Autodesk Inventor part; units mm, degrees
ref_plane "YZ Plane" through (0, 0, 0) normal (1, 0, 0) x (0, 1, 0)
ref_plane "XZ Plane" through (0, 0, 0) normal (0, 1, 0) x (-1, 0, 0)
ref_plane "XY Plane" through (0, 0, 0) normal (0, 0, 1) x (1, 0, 0)
sketch "スケッチ1" plane through (0, 0, 0) normal (0, 1, 0) x (-1, 0, 0)
  line L0 (-13.5, 21) -> (-19.5, 21)
  line L1 (-19.5, 21) -> (-19.5, 0)
  line L2 (-19.5, 0) -> (19.5, 0)
  line L3 (19.5, 0) -> (19.5, 21)
  line L4 (19.5, 21) -> (13.5, 21)
  line L5 (13.5, 21) -> (13.5, 47)
  line L6 (13.5, 47) -> (19.5, 47)
  line L7 (19.5, 47) -> (19.5, 53)
  line L8 (19.5, 53) -> (-19.5, 53)
  line L9 (-19.5, 53) -> (-19.5, 47)
  line L10 (-19.5, 47) -> (-13.5, 47)
  line L11 (-13.5, 47) -> (-13.5, 21)
  point P0 (0, 0)
  point P1 (0, 0)
  dimension "d5" = 39
  dimension "d6" = 27
  dimension "d8" = 26
  dimension "d16" = 6
  dimension "d43" = 53
  dimension "d44" = 39
extrude "Body" add sketch "スケッチ1" along normal blind 0.8
fillet "フィレット1" radius 1 6 edges at (19.5, 0.4, 53) (19.5, 0.4, 47) (19.5, 0.4, 21) (-19.5, 0.4, 21) (-19.5, 0.4, 53) (-19.5, 0.4, 47)
sketch "スケッチ6" plane through (0, 0, 0) normal (0, -1, 0) x (1, 0, 0)
  circle A0 centre (0, 18.2) radius 7.5
  line L0 (19.5, 0) -> (-19.5, 0)
  circle A1 centre (0, 18.2) radius 10
  point P0 (0, 0)
  point P1 (0, 0)
  dimension "d27" = 15
  dimension "d28" = 20
  dimension "d31" = 18.2
extrude "押し出し4" cut sketch "スケッチ6" against normal through all contours A0
sketch "スケッチ7" plane through (0, 0.8, 0) normal (0, 1, 0) x (1, 0, 0)
  spline S0 degree 5 poles (0, 0) (-0.3117, -0.0168) (-0.9317, -0.0488) (-1.8515, -0.0923) (-3.0577, -0.1409) (-4.5307, -0.1873) (-5.9672, -0.223) (-7.3645, -0.2562) (-8.7185, -0.3001) (-10.0237, -0.3761) (-11.2732, -0.5129) (-12.4592, -0.7408) (-13.5734, -1.0876) (-14.6076, -1.5729) (-15.5546, -2.2027) (-16.4082, -2.9673) (-17.1633, -3.8489) (-17.8162, -4.8254) (-18.3648, -5.8755) (-18.8088, -6.9843) (-19.1492, -8.1424) (-19.3399, -9.1044) (-19.4375, -9.8448) (-19.4825, -10.3469) (-19.5, -10.6) knots 0 0 0 0 0 0 0.05 0.1 0.15 0.2 0.25 0.3 0.35 0.4 0.45 0.5 0.55 0.6 0.65 0.7 0.75 0.8 0.85 0.9 0.95 1 1 1 1 1 1
  spline S1 degree 5 poles (19.5, -10.6) (19.4825, -10.3469) (19.4375, -9.8448) (19.3399, -9.1043) (19.1492, -8.1424) (18.8088, -6.9842) (18.3648, -5.8755) (17.8162, -4.8253) (17.1633, -3.8489) (16.4081, -2.9673) (15.5546, -2.2027) (14.6076, -1.5729) (13.5734, -1.0876) (12.4592, -0.7408) (11.2732, -0.5129) (10.0237, -0.3762) (8.7184, -0.3002) (7.3644, -0.2562) (5.9671, -0.2231) (4.5306, -0.1873) (3.0577, -0.141) (1.8515, -0.0923) (0.9316, -0.0489) (0.3116, -0.0169) (0, 0) knots -1 -1 -1 -1 -1 -1 -0.95 -0.9 -0.85 -0.8 -0.75 -0.7 -0.65 -0.6 -0.55 -0.5 -0.45 -0.4 -0.35 -0.3 -0.25 -0.2 -0.15 -0.1 -0.05 0 0 0 0 0 0
  line L0 (19.5, -10.6) -> (19.5, -53)
  line L1 (19.5, -53) -> (-19.5, -53)
  line L2 (-19.5, -53) -> (-19.5, -10.6)
  line L3 (-18.5, -53) -> (18.5, -53)
  line L4 (19.5, 0) -> (-19.5, 0)
  point P0 (0, -53)
  dimension "d40" = 53
  dimension "d45" = 39
  dimension "d47" = 10.6
extrude "押し出し5" cut sketch "スケッチ7" against normal through all keep common part
sketch "スケッチ9" plane through (0, 0, 0) normal (0, -1, 0) x (1, 0, 0)
  circle A0 centre (-11.5, 47) radius 1
  circle A1 centre (-11.5, 47) radius 1
  circle A2 centre (-11.5, 18) radius 1
  line L0 (0, 0) -> (0, 53)
  circle A3 centre (11.5, 47) radius 1
  circle A4 centre (11.5, 47) radius 1
  circle A5 centre (11.5, 18) radius 1
  line L1 (-18.5, 53) -> (18.5, 53)
  circle A6 centre (0, 18.2) radius 7.5
  line L2 (19.5, 20) -> (19.5, 10.6)
  arc A7 (19.5, 20) -> (18.5, 21) centre (18.5, 20) ccw
  line L3 (13.5, 21) -> (18.5, 21)
  line L4 (13.5, 47) -> (13.5, 21)
  line L5 (18.5, 47) -> (13.5, 47)
  arc A8 (18.5, 47) -> (19.5, 48) centre (18.5, 48) ccw
  line L6 (19.5, 52) -> (19.5, 48)
  arc A9 (19.5, 52) -> (18.5, 53) centre (18.5, 52) ccw
  line L7 (-18.5, 53) -> (18.5, 53)
  arc A10 (-18.5, 53) -> (-19.5, 52) centre (-18.5, 52) ccw
  line L8 (-19.5, 48) -> (-19.5, 52)
  arc A11 (-19.5, 48) -> (-18.5, 47) centre (-18.5, 48) ccw
  line L9 (-13.5, 47) -> (-18.5, 47)
  line L10 (-13.5, 21) -> (-13.5, 47)
  line L11 (-18.5, 21) -> (-13.5, 21)
  arc A12 (-18.5, 21) -> (-19.5, 20) centre (-18.5, 20) ccw
  line L12 (-19.5, 10.6) -> (-19.5, 20)
  dimension "d52" = 2
  dimension "d53" = 29
  dimension "d55" = 2
extrude "押し出し7" cut sketch "スケッチ9" against normal through all contours A0 | A2 | A3 | A5
ref_plane "作業平面1" through (13.5, 0, 34) normal (0, 0, -1) x (-1, 0, 0)
properties part number "MainBoard"
Work out the finished part from the listing and answer in its coordinate system (mm). A direction names the side the tool comes from. Coordinates: 2 decimals unless noted, no trailing zeros. Loops run counter-clockwise (first coordinate to the right, second up) from the corner with the lowest first, then second, coordinate; pieces in that order, holes last. Notation, with made-up numbers: (-29, 42) -> (-11, 42) arc R6 cw to (-11, 53) -> close; hole circle Ø7 at (71.25, 40.25). An arc over 180 degrees is marked (long way). Answer as CSV lines item,"result".
1) Straight lines are drawn through the part: probe 1 along Z at (x, y) = (0, 0.25); probe 2 along Z at (x, y) = (-11.5, 0.4); probe 3 along X at (y, z) = (0.6, 11.5). For each, find the intervals that lie inside material, in ascending order.
A:
probe 1,"z = 0 to 10.7, 25.7 to 53"
probe 2,"z = 0.57 to 17, 19 to 46, 48 to 53"
probe 3,"x = -19.5 to -3.37, 3.37 to 19.5"
2) For a pull along Z with two mould halves and no side action, classify faces 4 (the face through (0, 0.8, 27)), 5 (the face through (-11.63, 0.39, 47.99)), 6 (the face through (19.199, 0.406, 52.715)) as released by +Z, released by -Z, zero draft, split by the parting line, or undercut.
A:
face 4,"zero draft"
face 5,"undercut"
face 6,"released by +Z"
3) The part is cut by section A-A (y = 0.15). State how many separate pieces and enclosed holes the cut face has, and give its area (3 significant figures).
A:
separate pieces,"1"
enclosed holes,"5"
area,"1,510 mm²"
4) For faces 1 (the face through (-1.63, 0.39, 10.88)), 2 (the face through (-19.199, 0.406, 47.285)), 3 (the face through (19.215, 0.406, 47.301)), determine the directions among +Z, -Z, +X, -X, +Y, -Y from which every point of the face is accessible in a straight line to the end or side of a thin tool.
A:
face 1,"+Y, -Y"
face 2,"-X, +Y, -Y"
face 3,"+X, +Y, -Y"
5) The part is cut by section B-B (z = 35). Give the vertices of the cut face in (x, y), and give its area (3 significant figures).
A:
outline,"(-13.5, 0) -> (13.5, 0) -> (13.5, 0.8) -> (-13.5, 0.8) -> close"
area,"21.6 mm²"
